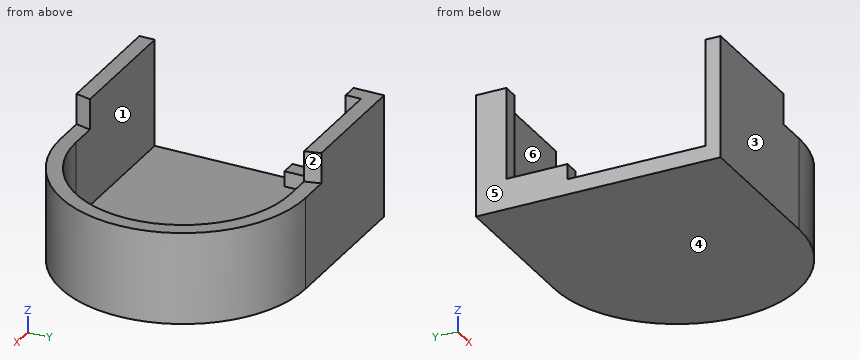
Autodesk Inventor part; units mm, degrees
ref_plane "YZ Plane" through (0, 0, 0) normal (1, 0, 0) x (0, 1, 0)
ref_plane "XZ Plane" through (0, 0, 0) normal (0, 1, 0) x (-1, 0, 0)
ref_plane "XY Plane" through (0, 0, 0) normal (0, 0, 1) x (1, 0, 0)
sketch "Sketch1" plane through (0, 0, 0) normal (0, 0, 1) x (1, 0, 0)
  line L0 (0, 0) -> (50, 0)
  line L1 (50, 0) -> (50, 80) construction
  line L2 (50, 80) -> (0, 80)
  line L3 (0, 80) -> (0, 0)
  circle A0 centre (50, 40) radius 40 construction
  arc A1 (50, 0) -> (50, 80) centre (50, 40) ccw
  dimension "d0" = 50
  dimension "d1" = 80
  dimension "d2" = 80
extrude "Extrusion1" add sketch "Sketch1" along normal blind 40
sketch "Sketch2" plane through (0, 0, 40) normal (0, 0, 1) x (1, 0, 0)
  line L0 (50, 80) -> (0, 80)
  arc A0 (50, 0) -> (50, 80) centre (50, 40) ccw
  line L1 (0, 0) -> (50, 0)
  line L2 (0, 75) -> (50, 75)
  arc A1 (50, 5) -> (50, 75) centre (50, 40) ccw
  line L3 (50, 5) -> (0, 5)
  line L4 (0, 75) -> (0, 5)
  line L5 (0, 80) -> (0, 0)
  dimension "d5" = 5
extrude "Extrusion2" cut sketch "Sketch2" against normal blind 35 contours L2 A1 L3 L4
sketch "Sketch3" plane through (0, 0, 0) normal (-1, 0, 0) x (0, 0, 1)
  line L0 (0, 80) -> (0, 0)
  line L1 (40, 75) -> (40, 5)
  line L2 (0, 80) -> (40, 80)
  line L3 (40, 80) -> (40, 70)
  line L4 (40, 70) -> (0, 70)
  line L5 (0, 70) -> (0, 80)
  line L6 (0, 80) -> (10, 80)
  line L7 (10, 80) -> (10, 50)
  line L8 (10, 50) -> (0, 50)
  line L9 (0, 50) -> (0, 80)
  line L10 (0, 0) -> (40, 0)
  dimension "d8" = 10
  dimension "d9" = 10
  dimension "d10" = 50
extrude "Extrusion3" add sketch "Sketch3" against normal blind 5
sketch "Sketch4" plane through (0, 0, 40) normal (0, 0, 1) x (1, 0, 0)
  line L0 (50, 80) -> (50, 0)
  arc A0 (50, 0) -> (50, 80) centre (50, 40) ccw
  arc A1 (50, 0) -> (50, 80) centre (50, 40) ccw
  arc A2 (50, 0) -> (50, 80) centre (50, 40) ccw
  line L1 (50, 40) -> (40, 80)
  line L2 (50, 80) -> (0, 80)
  line L3 (40, 80) -> (50, 80)
  line L4 (50, 40) -> (40, 0)
  line L5 (0, 0) -> (50, 0)
  line L6 (40, 0) -> (50, 0)
  dimension "d15" = 10
extrude "Extrusion4" cut sketch "Sketch4" against normal blind 10
properties part number "FA004" material "ABS Plastic"
Could you check a few things on this model? Use its own coordinates, in mm. Face numbers are marked on the shaded views. A direction names the side the tool comes from. Coordinates: 2 decimals unless noted, no trailing zeros. Write each loop counter-clockwise with the first axis right and the second up, starting at its lowest first coordinate (ties: lowest second). Pieces come first, ordered by that corner, then holes. Notation, with made-up numbers: (-7, 58.5) -> (36, 58.5) arc R22 ccw to (36, 81.5) -> close; hole circle Ø5 at (29.25, 6). An arc over 180 degrees is marked (long way). One line per question, with ' | ' between items. Start each with the question number.
1. If we section it at C-C (y = 40): Please give me the cut outline in (x, z), and give its area (3 significant figures).
2. If we section it at B-B (x = 47): Please give me the cut outline in (y, z).
3. Thinking about a two-plate mould opening in Y: for the marked faces 1, 2, 3 and 4, which applies, pulls with the +Y half, pulls with the -Y half, needs draft (parallel to the pull), parting line crosses it, or undercut?
4. Will these pins go through, and if not, where does the flat tip stop? P1, Ø8, axis at y = 26, z = 15, coming from the -X side; P2, Ø5, axis at y = 64, z = 16.5, coming from the +X side; P3, Ø25, axis at x = 55, y = 36, coming from the +Z side.
5. If we section it at A-A (z = 36.5): Please give me the cut outline in (x, y), and give its area (3 significant figures).
6. Please list where these lines run through material, in increasing order: line 1 along Y through (x, z) = (47, 27); line 2 along Z through (x, y) = (57, 15.5); line 3 along Y through (x, z) = (78.5, 27.5).
7. For the marked faces 5 and 6, which set-ups out of +Z, -Z, +X, -X, +Y, -Y let a thin tool reach every point of the face, with its end or its side?
8. If we section it at D-D (z = 26.5): Please give me the cut outline in (x, y).
Return value:
1) outline: (0, 0) -> (90, 0) -> (90, 30) -> (85, 30) -> (85, 5) -> (0, 5) -> close | area: 575 mm²
2) outline: (0, 0) -> (80, 0) -> (80, 30) -> (75, 30) -> (75, 5) -> (5, 5) -> (5, 30) -> (0, 30) -> close
3) face 1: undercut | face 2: pulls with the +Y half | face 3: pulls with the -Y half | face 4: needs draft
4) P1: stops at x = 80.02 | P2: stops at x = 83.73 | P3: stops at z = 5
5) outline: (0, 0) -> (40, 0) -> (41.25, 5) -> (0, 5) -> close; (0, 70) -> (5, 70) -> (5, 75) -> (41.25, 75) -> (40, 80) -> (0, 80) -> close | area: 431 mm²
6) line 1: y = 0 to 5, 75 to 80 | line 2: z = 0 to 5 | line 3: y = 11.93 to 19.68, 60.32 to 68.07
7) face 5: +Z, -Z, -X, +Y, -Y | face 6: +Z
8) outline: (0, 0) -> (50, 0) arc R40 ccw to (50, 80) -> (0, 80) -> (0, 70) -> (5, 70) -> (5, 75) -> (50, 75) arc R35 cw to (50, 5) -> (0, 5) -> close
